Solid Edge part; units mm, degrees
sketch "Sketch1" plane through (0, 0, 0) normal (0, 0, 1) x (1, 0, 0)
  line L0 (-68.5, -40) -> (68.5, -40)
  line L1 (68.5, -40) -> (68.5, 40)
  line L2 (68.5, 40) -> (-68.5, 40)
  line L3 (-68.5, 40) -> (-68.5, -40)
  dimension "D1" = 68.5
  dimension "D2" = 68.5
extrude "Protrusion1" add sketch "Sketch1" along normal mid plane 27
sketch "Sketch2" plane through (0, 0, 13.5) normal (0, 0, 1) x (1, 0, 0)
  line L0 (-68.5, 40) -> (11.5, 40)
  line L1 (11.5, 40) -> (11.5, 28)
  line L2 (11.5, 28) -> (-68.5, 28)
  line L3 (-68.5, 28) -> (-68.5, 40)
  dimension "D1" = 68.5
  dimension "D2" = 11.5
extrude "Cutout1" cut sketch "Sketch2" against normal up to next
sketch "Sketch3" plane through (0, 0, 13.5) normal (0, 0, 1) x (1, 0, 0)
  line L0 (-68.5, -40) -> (11.5, -40)
  line L1 (11.5, -40) -> (11.5, -18)
  line L2 (11.5, -18) -> (-68.5, -18)
  line L3 (-68.5, -18) -> (-68.5, -40)
  dimension "D1" = 11.5
  dimension "D2" = 11.5
extrude "Cutout2" cut sketch "Sketch3" against normal up to next
sketch "Sketch4" plane through (0, 0, -13.5) normal (0, 0, -1) x (1, 0, 0)
  line L0 (68.5, 40) -> (11.5, 40)
  line L1 (11.5, 40) -> (11.5, 10)
  line L2 (11.5, 10) -> (68.5, 10)
  line L3 (68.5, 10) -> (68.5, 40)
  dimension "D1" = 11.5
  dimension "D2" = 68.5
extrude "Extrusionsausschnitt_3" cut sketch "Sketch4" against normal blind 15.56
sketch "Sketch5" plane through (0, 0, 13.5) normal (0, 0, 1) x (1, 0, 0)
  line L0 (11.5, 40) -> (68.5, 40)
  line L1 (68.5, 40) -> (68.5, -40)
  line L2 (68.5, -40) -> (11.5, -40)
  line L3 (11.5, -40) -> (11.5, 40)
extrude "Extrusionsausprägung_4" add sketch "Sketch5" along normal blind 6
sketch "Sketch6" plane through (40, -40, 10.78) normal (0, -1, 0) x (1, 0, 0)
  line L0 (-28.5, 8.72) -> (28.5, 8.72)
  line L1 (28.5, 8.72) -> (28.5, -8.72)
  line L2 (28.5, -8.72) -> (-28.5, -8.72)
  line L3 (-28.5, -8.72) -> (-28.5, 8.72)
extrude "Extrusionsausprägung_13" add sketch "Sketch6" along normal blind 3
hole "Bohrung_6" at (-64.1, -13.6, -13.5) direction (0, 0, 1) diameter 6.4 depth 16
hole "Hole1" at (7.1, -13.6, -13.5) direction (0, 0, 1) diameter 6.4 depth 16
hole "Hole2" at (-64.1, 23.6, -13.5) direction (0, 0, 1) diameter 6.4 depth 16
hole "Hole3" at (15.9, 35.6, -13.5) direction (0, 0, 1) diameter 6.4 depth 16
hole "Hole4" at (64.1, 35.6, -13.5) direction (0, 0, 1) diameter 6.4 depth 16
hole "Bohrung_11" at (15.9, -35.6, 2.06) direction (0, 0, 1) diameter 6.4 depth 16
hole "Hole5" at (57.1, -14.4, 2.06) direction (0, 0, 1) diameter 6.4 depth 16
sketch "Sketch7" plane through (68.5, 0, 3) normal (1, 0, 0) x (0, 0, 1)
  circle A0 centre (-0.94, 26.91) radius 6.5
  dimension "D1" = 0.94
extrude "Extrusionsausschnitt_7" cut sketch "Sketch7" against normal blind 5.05
sketch "Sketch8" plane through (68.5, 0, 3) normal (1, 0, 0) x (0, -1, 0)
  circle A0 centre (-5, 16.5) radius 10.5
  dimension "D1" = 5
extrude "Extrusionsausschnitt_8" cut sketch "Sketch8" against normal blind 8
sketch "Sketch9" plane through (-27.5, 28, 0) normal (0, 1, 0) x (1, 0, 0)
  circle A0 centre (-4.11, 13.5) radius 13
extrude "Extrusionsausschnitt_9" cut sketch "Sketch9" against normal blind 95
hole "Bohrung_19" at (-64.1, 23.6, 13.5) direction (0, 0, -1) diameter 5.6 depth 10
hole "Hole6" at (-64.1, -13.6, 13.5) direction (0, 0, -1) diameter 5.6 depth 10
hole "Hole7" at (7.1, -13.6, 13.5) direction (0, 0, -1) diameter 5.6 depth 10
hole "Hole8" at (7.1, 23.6, 13.5) direction (0, 0, -1) diameter 5.6 depth 10
sketch "Sketch10" plane through (-27.5, 5, 13.5) normal (0, 0, 1) x (1, 0, 0)
  line L0 (-31.61, 17.11) -> (23.39, 17.11)
  line L1 (23.39, 17.11) -> (23.39, -0.89)
  line L2 (23.39, -0.89) -> (-31.61, -0.89)
  line L3 (-31.61, -0.89) -> (-31.61, 17.11)
  dimension "D1" = 23.39
  dimension "D2" = 31.61
extrude "Extrusionsausprägung_11" add sketch "Sketch10" along normal blind 4
fillet "Verrundung_12" radius 1 8 edges at (-31.61, 4.11, 13.5) (-59.11, 13.11, 13.5) (-59.11, 13.11, 17.5) (-31.61, 4.11, 17.5) (-31.61, 22.11, 13.5) (-31.61, 22.11, 17.5) (-4.11, 13.11, 13.5) (-4.11, 13.11, 17.5)
sketch "Sketch11" plane through (24.945, 11, -13.5) normal (0, 0, -1) x (1, 0, 0)
  line L0 (-43.555, 29) -> (-45.055, 29)
  line L1 (-45.055, 29) -> (-45.055, 27.29)
  line L2 (-45.055, 27.29) -> (-43.555, 27.29)
  line L3 (-43.555, 27.29) -> (-43.555, 29)
  line L4 (-43.555, -17) -> (-45.055, -17)
  line L5 (-45.055, -17) -> (-45.055, -15.29)
  line L6 (-45.055, -15.29) -> (-43.555, -15.29)
  line L7 (-43.555, -15.29) -> (-43.555, -17)
revolve "Rotationsausprägung_1" add sketch "Sketch11" angle 180 about axis through (-31.61, -20.9276, -13.5) along (0, -1, 0)
sketch "Sketch12" plane through (-54.805, 5, -13.5) normal (0, 0, -1) x (0, -1, 0)
  line L0 (-16.29, -10.195) -> (-16.29, 5.305)
  line L1 (-16.29, 5.305) -> (-2.29, 5.305)
  line L2 (-2.29, 5.305) -> (-2.29, -3.195)
  line L3 (-2.29, -3.195) -> (9.29, -3.195)
  line L4 (9.29, -3.195) -> (16.29, -10.195)
  line L5 (16.29, -10.195) -> (-16.29, -10.195)
  dimension "D1" = 16.29
  dimension "D2" = 16.29
revolve "RevolvedCutout1" cut sketch "Sketch12" angle 360 about axis through (-31.61, 30.2296, -13.5) along (0, -1, 0)
sketch "Sketch13" plane through (40, -26.5, 2.06) normal (0, 0, -1) x (-1, 0, 0)
  line L0 (17.8, -0.41) -> (17.8, 5.09)
  line L1 (17.8, 5.09) -> (14.8, 5.09)
  line L2 (14.8, 5.09) -> (14.8, 6.09)
  line L3 (14.8, 6.09) -> (8.5, 6.09)
  line L4 (8.5, 6.09) -> (8.5, -0.41)
  line L5 (8.5, -0.41) -> (17.8, -0.41)
  dimension "D1" = 14.8
  dimension "D2" = 17.8
revolve "RevolvedCutout2" cut sketch "Sketch13" angle 360 about axis through (68.5, -26.91, 2.06) along (-1, 0, 0)
sketch "Sketch14" plane through (40, -26.5, 2.06) normal (0, 0, -1) x (-1, 0, 0)
  line L0 (8.5, -0.41) -> (8.5, 12.59)
  line L1 (8.5, 12.59) -> (-6.5, 12.59)
  line L2 (-6.5, 12.59) -> (-6.5, 5.09)
  line L3 (-6.5, 5.09) -> (-23.45, 5.09)
  line L4 (-23.45, 5.09) -> (-23.45, -0.41)
  line L5 (-23.45, -0.41) -> (8.5, -0.41)
  dimension "D1" = 8.5
revolve "RevolvedCutout3" cut sketch "Sketch14" angle 360 about axis through (68.5, -26.91, 2.06) along (-1, 0, 0)
sketch "Sketch15" plane through (24.195, 11, -13.5) normal (0, 0, -1) x (-1, 0, 0)
  line L0 (-27.355, -6) -> (-22.255, -6)
  line L1 (-22.255, -6) -> (-22.255, 6)
  line L2 (-22.255, 6) -> (-27.355, 6)
  line L3 (-27.355, 6) -> (-27.355, -6)
  dimension "D1" = 22.255
revolve "RevolvedCutout4" cut sketch "Sketch15" angle 360 about axis through (68.5, 5, -13.5) along (-1, 0, 0)
sketch "Sketch16" plane through (24.195, 11, -13.5) normal (0, 0, -1) x (-1, 0, 0)
  line L0 (-22.255, -6) -> (-22.255, 22.5)
  line L1 (-22.255, 22.5) -> (-7.305, 22.5)
  line L2 (-7.305, 22.5) -> (-7.305, -6)
  line L3 (-7.305, -6) -> (-22.255, -6)
  dimension "D1" = 22.255
revolve "RevolvedCutout5" cut sketch "Sketch16" angle 360 about axis through (68.5, 5, -13.5) along (-1, 0, 0)
sketch "Sketch17" plane through (24.195, 11, -13.5) normal (0, 0, -1) x (-1, 0, 0)
  line L0 (10.145, -6) -> (15.245, -6)
  line L1 (15.245, -6) -> (15.245, 6)
  line L2 (15.245, 6) -> (10.145, 6)
  line L3 (10.145, 6) -> (10.145, -6)
  line L4 (20.145, -6) -> (25.245, -6)
  line L5 (25.245, -6) -> (25.245, 6)
  line L6 (25.245, 6) -> (20.145, 6)
  line L7 (20.145, 6) -> (20.145, -6)
  dimension "D1" = 15.245
revolve "RevolvedCutout6" cut sketch "Sketch17" angle 360 about axis through (68.5, 5, -13.5) along (-1, 0, 0)
sketch "Sketch18" plane through (24.195, 11, -13.5) normal (0, 0, -1) x (-1, 0, 0)
  line L0 (-27.355, -6) -> (-27.355, 4.5)
  line L1 (-27.355, 4.5) -> (-36.305, 4.5)
  line L2 (-36.305, 4.5) -> (-36.305, -6)
  line L3 (-36.305, -6) -> (-27.355, -6)
revolve "RevolvedCutout7" cut sketch "Sketch18" angle 360 about axis through (68.5, 5, -13.5) along (-1, 0, 0)
sketch "Sketch19" plane through (24.195, 11, -13.5) normal (0, 0, -1) x (-1, 0, 0)
  line L0 (-7.305, -6) -> (-7.305, 12)
  line L1 (-7.305, 12) -> (10.145, 4.5)
  line L2 (10.145, 4.5) -> (10.145, -6)
  line L3 (10.145, -6) -> (-7.305, -6)
revolve "RevolvedCutout8" cut sketch "Sketch19" angle 360 about axis through (68.5, 5, -13.5) along (-1, 0, 0)
sketch "Sketch20" plane through (24.195, 11, -13.5) normal (0, 0, -1) x (-1, 0, 0)
  line L0 (15.245, -6) -> (20.145, -6)
  line L1 (20.145, -6) -> (20.145, 4.5)
  line L2 (20.145, 4.5) -> (15.245, 4.5)
  line L3 (15.245, 4.5) -> (15.245, -6)
revolve "RevolvedCutout9" cut sketch "Sketch20" angle 360 about axis through (-1.05, 5, -13.5) along (1, 0, 0)
sketch "Sketch21" plane through (24.195, 11, -13.5) normal (0, 0, -1) x (-1, 0, 0)
  line L0 (25.245, -6) -> (25.245, -16.5)
  line L1 (25.245, -16.5) -> (29.245, -16.5)
  line L2 (29.245, -16.5) -> (38.245, -13.5)
  line L3 (38.245, -13.5) -> (38.245, -6)
  line L4 (38.245, -6) -> (25.245, -6)
  dimension "D1" = 25.245
revolve "RevolvedCutout10" cut sketch "Sketch21" angle 360 about axis through (14.05, 5, -13.5) along (-1, 0, 0)
sketch "Sketch22" plane through (68.5, -1.5, 3) normal (1, 0, 0) x (0, 0, -1)
  line L0 (16.5, 17) -> (16.5, 41.5)
  line L1 (16.5, 41.5) -> (-16.5, 41.5)
  line L2 (-16.5, 41.5) -> (-16.5, -41.5)
  line L3 (-16.5, -41.5) -> (0.94, -41.5)
  line L4 (0.94, -41.5) -> (0.94, -31.41)
  line L5 (0.94, -19.41) -> (0.94, -8.5)
  line L6 (0.94, -8.5) -> (16.5, -8.5)
  line L7 (16.5, -8.5) -> (16.5, -4)
  arc A0 (16.5, 17) -> (16.5, -4) centre (16.5, 6.5) ccw
  arc A1 (0.94, -31.41) -> (0.94, -19.41) centre (0.94, -25.41) cw
extrude "Extrusionsausprägung_14" add sketch "Sketch22" along normal blind 1
properties part number "3" material "Polykarbonat"
Geometry: final body of the model. Coordinates: model frame, mm. A direction names the side the tool comes from. Round coordinates to 2 decimals unless told otherwise and drop trailing zeros. Write each loop counter-clockwise with the first axis right and the second up, starting at its lowest first coordinate (ties: lowest second). Pieces come first, ordered by that corner, then holes. Notation, with made-up numbers: (54, 32) -> (104, 32) arc R17 cw to (104, 37) -> close; hole circle Ø11 at (-37.5, -10). An arc over 180 degrees is marked (long way). Return JSON: item names as keys, results as strings.
Q1. Section B-B on x = -64.1. Return the cut outline in (y, z).
From the geometry:
{"outline": "(-18, -13.5) -> (-16.8, -13.5) -> (-16.8, 2.5) -> (-10.4, 2.5) -> (-10.4, -13.5) -> (20.4, -13.5) -> (20.4, 2.5) -> (26.8, 2.5) -> (26.8, -13.5) -> (28, -13.5) -> (28, 13.5) -> (26.4, 13.5) -> (26.4, 3.5) -> (20.8, 3.5) -> (20.8, 13.5) -> (-10.8, 13.5) -> (-10.8, 3.5) -> (-16.4, 3.5) -> (-16.4, 13.5) -> (-18, 13.5) -> close"}
Q2. Mould query, pull axis Y, two halves, no side actions, for faces 4 (the cylindrical face through (66.01, -26.77, 8.56)), 5 (the conical face through (-9.06, -0.35, -6.06)), 6 (the flat face through (41, -43, 11)), 7 (the flat face through (69.5, 7, 6)). Classes: +Y half, -Y half, draft (parallel to the pull), parting line (faces both ways), or undercut.
From the geometry:
{"face 4": "undercut", "face 5": "undercut", "face 6": "-Y half", "face 7": "draft"}
Q3. Section A-A on y = 35.6. Return the cut outline in (x, z).
From the geometry:
{"outline": "(11.5, -13.5) -> (12.7, -13.5) -> (12.7, 2.5) -> (19.1, 2.5) -> (19.1, -13.5) -> (60.9, -13.5) -> (60.9, 2.5) -> (67.3, 2.5) -> (67.3, -13.5) -> (69.5, -13.5) -> (69.5, 19.5) -> (11.5, 19.5) -> close"}
Q4. First-contact query: pin 1 Ø5 at (x, y) = (-23.5, 1) entering from -Z; pin 2 Ø6 at (x, y) = (7.5, 23) entering from +Z; pin 3 Ø6 at (x, y) = (-64.1, -13.6) entering from -Z. Flat tips, straight axial feed; report the tip coordinate or a pass-through.
From the geometry:
{"pin 1": "z = 3.45", "pin 2": "z = 13.5", "pin 3": "z = 2.5"}
Q5. Set-up query: faces 1 (the cylindrical face through (13.74, -37.96, 10.17)), 2 (the flat face through (-64, -14, 3.5)), 3 (the flat face through (28, -34, 2.06)). Return all of +Z, -Z, +X, -X, +Y, -Y with unobstructed straight access to the full face (end or side cutting, diameter ignored); none if empty.
From the geometry:
{"face 1": "-Z", "face 2": "+Z", "face 3": "-Z, +X, -Y"}
Q6. Ray query, line 1 (Y direction, x = 7.1, z = 11.25); line 2 (Y direction, x = -59, z = -9); line 3 (X direction, y = 0, z = -2). Return the intervals inside material, ascending.
From the geometry:
{"line 1": "-18 to -16.4, -10.8 to 20.8, 26.4 to 28", "line 2": "-18 to 7.29, 21.29 to 28", "line 3": "-68.5 to -47.97, -15.25 to 18.8, 46.45 to 69.5"}
Q7. Section D-D on x = 29. Return the cut outline in (y, z), and give its area (3 significant figures).
From the geometry:
{"outline": "(-43, 2.06) -> (-33.41, 2.06) arc R6.5 cw to (-20.41, 2.06) -> (-10, 2.06) -> (-10, -5.66) arc R16.93 cw to (21.93, -13.5) -> (40, -13.5) -> (40, 19.5) -> (-43, 19.5) -> close", "area": "1,720 mm2"}
Q8. Section C-C on z = -10.5. Give the number of separate pieces and of enclosed holes in the cut face, and give its area (3 significant figures).
From the geometry:
{"separate pieces": "4", "enclosed holes": "5", "area": "2,530 mm2"}
